from build123d import *

# Parameters (mm, degrees)
SKETCH1_W             = 51.5
SKETCH1_H             = 2.5
BOSS_EXTRUDE1_DEPTH   = 9
BOSS_EXTRUDE1_2_DEPTH = 9
SKETCH2_W             = 52.5
SKETCH2_H             = 26.5
BOSS_EXTRUDE2_DEPTH   = 1.6
SKETCH3_W             = 29.4
SKETCH3_H             = 26.3
BOSS_EXTRUDE3_DEPTH   = 1.9
BOSS_EXTRUDE4_DEPTH   = 2.1
SKETCH5_W             = 1.9
SKETCH5_H             = 1.9
BOSS_EXTRUDE5_DEPTH   = 3


with BuildPart() as part:
    # Sketch1 → Boss-Extrude1 (new body)
    with BuildSketch(Plane(origin=(0, 0, 0), x_dir=(1, 0, 0), z_dir=(0, 1, 0))):
        with Locations((0, 8.875)):
            Rectangle(SKETCH1_W, SKETCH1_H)
    extrude(amount=BOSS_EXTRUDE1_DEPTH)



with BuildPart() as body_2:
    # Sketch1 → Boss-Extrude1 2 (new body)
    with BuildSketch(Plane(origin=(0, 0, 0), x_dir=(1, 0, 0), z_dir=(0, 1, 0))):
        with Locations((0, -8.875)):
            Rectangle(SKETCH1_W, SKETCH1_H)
    extrude(amount=BOSS_EXTRUDE1_2_DEPTH)


with BuildPart() as part_1:
    add(part.part)

    add(body_2.part)  # Boss-Extrude2 merges body 2
    # Sketch2 → Boss-Extrude2 (add)
    with BuildSketch(Plane(origin=(0, 9, 0), x_dir=(1, 0, 0), z_dir=(0, 1, 0))):
        Rectangle(SKETCH2_W, SKETCH2_H)
    extrude(amount=BOSS_EXTRUDE2_DEPTH)

    # Sketch3 → Boss-Extrude3 (add)
    with BuildSketch(Plane(origin=(0, 10.6, 0), x_dir=(1, 0, 0), z_dir=(0, 1, 0))):
        with Locations((-1.45, 0)):
            Rectangle(SKETCH3_W, SKETCH3_H)
    extrude(amount=BOSS_EXTRUDE3_DEPTH)

    # Sketch4 → Boss-Extrude4 (add)
    with BuildSketch(Plane(origin=(0, 10.6, 0), x_dir=(1, 0, 0), z_dir=(0, 1, 0))):
        Polygon((24.982590181, 0), (19.75, -5.232590181), (14.517409819, 0), (19.75, 5.232590181), align=None)
    extrude(amount=BOSS_EXTRUDE4_DEPTH)

    # Sketch5 → Boss-Extrude5 (add)
    with BuildSketch(Plane(origin=(0, 12.7, 0), x_dir=(1, 0, 0), z_dir=(0, 1, 0))):
        with Locations((19.75, 0)):
            Rectangle(SKETCH5_W, SKETCH5_H)
    extrude(amount=BOSS_EXTRUDE5_DEPTH)


solid = part_1.part
Geometry: final body of the model. Coordinates: model frame, mm. A direction names the side the tool comes from. Give positions to 0.01 mm unless a question says otherwise; leave off trailing zeros. Write each loop counter-clockwise with the first axis right and the second up, starting at its lowest first coordinate (ties: lowest second). Pieces come first, ordered by that corner, then holes.
(1) Cut plane D-D, the plane y = 14.5. Return loops of the section in (x, z), then the cut area to 3 significant figures.
(2) Cut plane A-A, the plane y = 4.25. Return loops of the section in (x, z) (3 decimals).
(3) Cut plane B-B, the plane z = -7. Return loops of the section in (x, y), then the cut area to 3 significant figures.
(4) Mould query, pull axis Z, two halves, no side actions, for faces 1 (the flat face through (0, 4, -7.625)), 2 (the flat face through (0, 4, 7.625)), 3 (the flat face through (18.8, 14, 0)), 4 (the flat face through (-2, 12, -13.15)). Classes: released by +Z, released by -Z, zero draft, split by the parting line, or undercut.
(5) Ray query, line 1 (Z direction, x = 1, y = 1.75) (3 decimals); line 2 (Y direction, x = 14, z = -2.25); line 3 (Y direction, x = 3.5, z = 10.75). Return the intervals inside material, ascending.
(6) Access query for faces 5 (the flat face through (-2, 12.5, 0)), 6 (the flat face through (22.33, 11.64, -2.65)), 7 (the flat face through (20, 14, -0.95)), 8 (the flat face through (25.75, 4, 9)), 9 (the flat face through (0, 4, -10.125)). Directions: +Z, -Z, +X, -X, +Y, -Y. A direction counts if a zero-diameter tool reaches every point of the face in a straight line with its end or side. Return the directions, or none.
(7) Cut plane C-C, the plane x = -21.5. Return loops of the section in (y, z) (3 decimals), then the cut area to 3 significant figures.
(8) First-contact query: P1, Ø1.5, axis at y = 14, z = 0.5, coming from the +X side; P2, Ø3, axis at y = 3.5, z = -9.5, coming from the +X side; P3, Ø0.6, axis at x = 5.5, y = 11.5, coming from the +Z side. Flat tips, straight axial feed; report the tip coordinate or a pass-through.
Values follow:
1. outline: (18.8, -0.95) - (20.7, -0.95) - (20.7, 0.95) - (18.8, 0.95) - close
1. area: 3.61 mm2
2. outline: (-25.75, -10.125) - (25.75, -10.125) - (25.75, -7.625) - (-25.75, -7.625) - close; (-25.75, 7.625) - (25.75, 7.625) - (25.75, 10.125) - (-25.75, 10.125) - close
3. outline: (-26.25, 9) - (26.25, 9) - (26.25, 10.6) - (13.25, 10.6) - (13.25, 12.5) - (-16.15, 12.5) - (-16.15, 10.6) - (-26.25, 10.6) - close
3. area: 140 mm2
4. face 1: undercut
4. face 2: undercut
4. face 3: zero draft
4. face 4: released by -Z
5. line 1: z = -10.125 to -7.625, 7.625 to 10.125
5. line 2: y = 9 to 10.6
5. line 3: y = 9 to 12.5
6. face 5: +Z, -Z, -X, +Y
6. face 6: -Z, +X, +Y
6. face 7: -Z, +X, -X, +Y
6. face 8: +Z, -Z, +X, -Y
6. face 9: -Z, +X, -X, -Y
7. outline: (0, -10.125) - (9, -10.125) - (9, -13.25) - (10.6, -13.25) - (10.6, 13.25) - (9, 13.25) - (9, 10.125) - (0, 10.125) - (0, 7.625) - (9, 7.625) - (9, -7.625) - (0, -7.625) - close
7. area: 87.4 mm2
8. P1: stops at x = 20.7
8. P2: stops at x = 25.75
8. P3: stops at z = 13.15
